Geometry: final body of the model. Coordinates: model frame, mm. A direction names the side the tool comes from. Give positions to 0.01 mm unless a question says otherwise; leave off trailing zeros. Write each loop counter-clockwise with the first axis right and the second up, starting at its lowest first coordinate (ties: lowest second). Pieces come first, ordered by that corner, then holes.
Q1. Cut plane A-A on y = 14.5. Return the cut outline in (x, z).
Q2. Draft query along X for faces 3 (the face through (-118.311, 51.341, 5.985)), 4 (the face through (-101, 0, 0)), 5 (the face through (-77, 27.55, 0)), 6 (the face through (-80.25, 17.89, 0.65)). Return one class per face: pulls with the +X half, pulls with the -X half, needs draft (parallel to the pull), parting line crosses it, or undercut.
Q3. Cut plane C-C on y = 66. Return the cut outline in (x, z), plus the area to 3 significant figures.
Q4. Cut plane B-B on z = 0. Return the cut outline in (x, y), plus the area to 3 significant figures.
Q5. Reachability of faces 1 (the face through (-95, 104.14, 0)), 2 (the face through (-88.161, 4, 0)) from +Z, -Z, +X, -X, +Y, -Y: full face, straight path, thin tool, end or side. Return the list, or none.
Q6. Pin query (flat end, axial travel): pin 1 (4 mm diameter, centred on y = 6, z = 0.5, fed in from +X); pin 2 (3 mm diameter, centred on x = -76.5, z = -1, fed in from -Y); pin 3 (4 mm diameter, centred on y = 63, z = 5, fed in from +X). Return the tip coordinate at first contact, or that it passes through.
Q7. Line query: L1, parallel to Y at x = -80, z = -0.75; L2, parallel to Y at x = -87, z = -6; L3, parallel to X at y = 91, z = -3. Output: solid intervals per line, ascending.
```python
from build123d import *

# Parameters (mm, degrees)
BOSS_EXTRUDE1_DEPTH = 104.14
SKETCH3_R           = 4.75
CUT_EXTRUDE4_DEPTH  = 104.14
SKETCH4_W           = 19.05
SKETCH4_H           = 15.24
CUT_EXTRUDE5_DEPTH  = 8.5
SKETCH5_R           = 3
CUT_EXTRUDE6_DEPTH  = 19.05


with BuildPart() as part:
    # Sketch1 → Boss-Extrude1 (new body)
    with BuildSketch(Plane(origin=(0, 0, 0), x_dir=(1, 0, 0), z_dir=(0, 1, 0))):
        with BuildLine():
            Line((-113.595187486, 7.62), (-69.111187486, 7.62))
            ThreePointArc((-69.111187486, 7.62), (-69.5299981, 0), (-69.111187486, -7.62))
            Line((-69.111187486, -7.62), (-113.595187486, -7.62))
            ThreePointArc((-113.595187486, -7.62), (-121.215187486, 0), (-113.595187486, 7.62))
        make_face()
    extrude(amount=BOSS_EXTRUDE1_DEPTH)

    # Sketch3 → Cut-Extrude4 (cut)
    with BuildSketch(Plane(origin=(0, 104.14, 0), x_dir=(1, 0, 0), z_dir=(0, 1, 0))):
        with Locations((-116.578948711, 0)):
            Circle(SKETCH3_R)
    extrude(amount=-CUT_EXTRUDE4_DEPTH, mode=Mode.SUBTRACT)

    # Sketch4 → Cut-Extrude5 (cut)
    with BuildSketch(Plane.XZ):
        with Locations((-78.636187486, 0)):
            Rectangle(SKETCH4_W, SKETCH4_H)
    extrude(amount=-CUT_EXTRUDE5_DEPTH, mode=Mode.SUBTRACT)

    # Sketch5 → Cut-Extrude6 (cut)
    with BuildSketch(Plane.XZ.offset(-8.5)):
        with Locations(Location((-77.323071778, 0, 0), (0, 0, 270))):
            Circle(SKETCH5_R)
    extrude(amount=-CUT_EXTRUDE6_DEPTH, mode=Mode.SUBTRACT)


solid = part.part
```
Data:
1. outline: (-121.04, -1.64) arc R7.62 ccw to (-113.6, -7.62) - (-69.11, -7.62) arc R69.53 cw to (-69.11, 7.62) - (-113.6, 7.62) arc R7.62 ccw to (-121.04, 1.64) arc R4.75 cw (long way) to start; hole circle Ø6 at (-77.32, 0)
2. face 3: pulls with the -X half
2. face 4: needs draft
2. face 5: undercut
2. face 6: undercut
3. outline: (-121.04, -1.64) arc R7.62 ccw to (-113.6, -7.62) - (-69.11, -7.62) arc R69.53 cw to (-69.11, 7.62) - (-113.6, 7.62) arc R7.62 ccw to (-121.04, 1.64) arc R4.75 cw (long way) to start
3. area: 694 mm2
4. outline: (-111.83, 0) - (-88.16, 0) - (-88.16, 8.5) - (-80.32, 8.5) - (-80.32, 27.55) - (-74.32, 27.55) - (-74.32, 8.5) - (-69.53, 8.5) - (-69.53, 104.14) - (-111.83, 104.14) - close
4. area: 4,130 mm2
5. face 1: +Z, -Z, +X, -X, +Y
5. face 2: +Z, -Z, +X, -Y
6. pin 1: stops at x = -88.16
6. pin 2: stops at y = 27.55
6. pin 3: stops at x = -69.18
7. L1: y = 27.55 to 104.14
7. L2: y = 8.5 to 104.14
7. L3: x = -120.6 to -120.26, -112.9 to -69.47
